Autodesk Inventor part; units mm, degrees
ref_plane "YZ Plane" through (0, 0, 0) normal (1, 0, 0) x (0, 1, 0)
ref_plane "XZ Plane" through (0, 0, 0) normal (0, 1, 0) x (-1, 0, 0)
ref_plane "XY Plane" through (0, 0, 0) normal (0, 0, 1) x (1, 0, 0)
sketch "スケッチ1" plane through (0, 0, 0) normal (1, 0, 0) x (0, 1, 0)
  line L0 (-42.5, 0) -> (42.5, 0) construction
  circle A0 centre (-42.5, 0) radius 4
  circle A1 centre (-42.5, 0) radius 8 construction
  circle A2 centre (-42.5, 8) radius 1.05
  line L1 (-42.5, 8) -> (-42.5, 0) construction
  circle A3 centre (-48.1569, 5.6569) radius 1.05
  circle A4 centre (-50.5, 0) radius 1.05
  circle A5 centre (-48.1569, -5.6569) radius 1.05
  circle A6 centre (-42.5, -8) radius 1.05
  circle A7 centre (-36.8431, -5.6569) radius 1.05
  circle A8 centre (-34.5, 0) radius 1.05
  circle A9 centre (-36.8431, 5.6569) radius 1.05
  arc A10 (-45.6384, 10.02) -> (-36.4408, -8.5753) centre (-42.5, 0) ccw
  arc A11 (36.4408, -8.5753) -> (-36.4408, -8.5753) centre (0, -60.1481) ccw
  arc A12 (45.6384, 10.02) -> (-45.6384, 10.02) centre (0, -135.6923) ccw
  arc A13 (36.4408, -8.5753) -> (45.6384, 10.02) centre (42.5, 0) ccw
  circle A14 centre (42.5, 0) radius 4
  circle A15 centre (42.5, 0) radius 8 construction
  line L2 (42.5, 0) -> (42.5, 8) construction
  circle A16 centre (42.5, 8) radius 1.05
  circle A17 centre (36.8431, 5.6569) radius 1.05
  circle A18 centre (34.5, 0) radius 1.05
  circle A19 centre (36.8431, -5.6569) radius 1.05
  circle A20 centre (42.5, -8) radius 1.05
  circle A21 centre (48.1569, -5.6569) radius 1.05
  circle A22 centre (50.5, 0) radius 1.05
  circle A23 centre (48.1569, 5.6569) radius 1.05
  line L3 (25.1751, 11.8679) -> (10.853, 5.1036) construction
  circle A24 centre (25.1751, 11.8679) radius 1.3
  circle A25 centre (10.853, 5.1036) radius 1.3
  circle A26 centre (25.1751, 11.8679) radius 3 construction
  circle A27 centre (10.853, 5.1036) radius 3 construction
  circle A28 centre (-3.7289, 13.9535) radius 1.3
  circle A29 centre (-1.7302, 5.9774) radius 1.3
  line L4 (0, 3) -> (0, 0) construction
  line L5 (0, 17) -> (0, 3) construction
  line L6 (-3.7289, 13.9535) -> (-1.7302, 5.9774) construction
  circle A30 centre (-3.7289, 13.9535) radius 3 construction
  circle A31 centre (-1.7302, 5.9774) radius 3 construction
  line L7 (-42.5, 0) -> (-2.7295, 9.9655) construction
  line L8 (23.7036, 7.7857) -> (-3.3435, -4.8265) construction
  arc A32 (30.9737, 13.8255) -> (24.6107, -1.9932) centre (42.5, 0) ccw construction
  dimension "d1" = 16
  dimension "d0" = 8
  dimension "d2" = 2.1
  dimension "d5" = 360
  dimension "d7" = 85
  dimension "d8" = 10.5
  dimension "d9" = 2.1
  dimension "d12" = 360
  dimension "d14" = 3
  dimension "d16" = 2.6
  dimension "d17" = 6
  dimension "d30" = 14
  dimension "d35" = 41
  dimension "d36" = 15
  dimension "d39" = 25
  dimension "d40" = 18
extrude "押し出し1" add sketch "スケッチ1" along normal blind 2
chamfer "面取り1" distance 1 angle 45 4 edges at (2, 0, 17) (2, -51.9117, -4.6552) (2, 0, 3) (2, 51.9117, -4.6552)
sketch "スケッチ2" plane through (2, 0, 0) normal (1, 0, 0) x (0, 0, -1)
  circle A0 centre (-13.9535, -3.7289) radius 1.3 construction
  circle A1 centre (-5.9774, -1.7302) radius 1.3 construction
  arc A2 (8.5753, 36.4408) -> (8.5753, -36.4408) centre (60.1481, 0) ccw construction
  arc A3 (-10.02, 45.6384) -> (-10.02, -45.6384) centre (135.6923, 0) ccw construction
  line L0 (-5.9774, -1.7302) -> (60.1481, 0) construction
  line L1 (-13.9535, -3.7289) -> (135.6923, 0) construction
  line L2 (-13.9535, -3.7289) -> (-16.9526, -3.8036) construction
  arc A4 (-13.8863, -6.428) -> (-14.0208, -1.0297) centre (-13.9535, -3.7289) ccw
  arc A5 (-6.048, 0.9689) -> (-5.9067, -4.4293) centre (-5.9774, -1.7302) ccw
  line L3 (-5.9067, -4.4293) -> (-2.85, -4.3493)
  line L4 (-6.048, 0.9689) -> (-2.9913, 1.0488)
  line L5 (-14.0208, -1.0297) -> (-16.996, -1.1038)
  line L6 (-13.8863, -6.428) -> (-16.8615, -6.5021)
  arc A6 (-16.996, -1.1038) -> (-16.8615, -6.5021) centre (135.6923, 0) ccw
  arc A7 (-2.9913, 1.0488) -> (-2.85, -4.3493) centre (60.1481, 0) ccw
  arc A8 (-12.3219, 22.5135) -> (-11.4138, 27.8366) centre (-11.8679, 25.1751) ccw
  arc A9 (-4.6606, 13.5165) -> (-5.5466, 8.1896) centre (-5.1036, 10.853) ccw
  line L7 (-4.6606, 13.5165) -> (-1.6443, 13.0148)
  line L8 (-5.5466, 8.1896) -> (-2.5303, 7.6879)
  line L9 (-12.3219, 22.5135) -> (-15.2557, 23.014)
  line L10 (-11.4138, 27.8366) -> (-14.3475, 28.3371)
  arc A10 (-14.3475, 28.3371) -> (-15.2557, 23.014) centre (135.6923, 0) ccw
  arc A11 (-1.6443, 13.0148) -> (-2.5303, 7.6879) centre (60.1481, 0) ccw
  circle A12 centre (-5.1036, 10.853) radius 1.3 construction
  circle A13 centre (-11.8679, 25.1751) radius 1.3 construction
  line L11 (-11.8679, 25.1751) -> (135.6923, 0) construction
  line L12 (60.1481, 0) -> (-5.1036, 10.853) construction
  point P0 (0, 0)
  dimension "d25" = 5.4
extrude "押し出し2" cut sketch "スケッチ2" against normal blind 1
properties part number "side_frame"
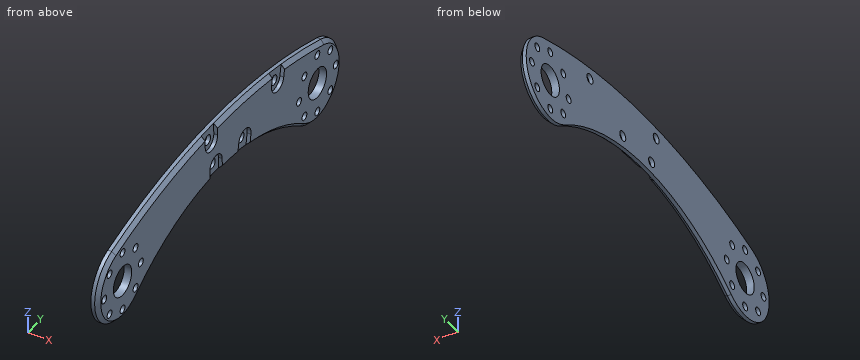
Source: CAD feature listing. Evaluate the final solid. Frame: model axes, mm. Coordinates: 2 decimals unless noted, no trailing zeros. Answer as CSV lines item,"result".
1. Section A-A (x = 0.6). Count the separate pieces of the cut face and the enclosed holes in it, then the cut area to 3 significant figures.
Established:
separate pieces,"1"
enclosed holes,"22"
area,"1,620 mm2"
2. Ray query, line 1 (Y direction, x = 0.4, z = 6.5); line 2 (Y direction, x = 1.05, z = -7.75); line 3 (Z direction, x = 0.45, y = 42). Return the intervals inside material, ascending.
Established:
line 1,"y = -50.75 to -48.78, -47.53 to -37.47, -36.22 to -2.92, -0.54 to 36.22, 37.47 to 47.53, 48.78 to 50.75"
line 2,"y = -49.51 to -43.52, -41.48 to -35.33, 35.33 to 41.48, 43.52 to 49.51"
line 3,"z = -10.49 to -8.92, -7.08 to -3.97, 3.97 to 7.08, 8.92 to 11.11"
3. Contact query for a flat-ended pin moving along its axis: pin 1 (5 mm diameter, centred on y = -3, z = 0.5, fed in from +X). Output: stop coordinate, or through.
Established:
pin 1,"stops at x = 1"
